The model under review builds one solid part; all positions refer to its coordinate system, in mm. Face numbers are marked on the shaded views. A direction names the side the tool comes from. Round coordinates to 2 decimals unless told otherwise and drop trailing zeros. Write each loop counter-clockwise with the first axis right and the second up, starting at its lowest first coordinate (ties: lowest second). Pieces come first, ordered by that corner, then holes.
Item 1: To check wall thickness, follow L1, parallel to X at y = 1.9, z = 3.5; L2, parallel to X at y = 0.6, z = -4.5; L3, parallel to X at y = 4.4, z = 0. State the ranges of each line that lie inside material, in increasing order.
Item 2: Clearance check with flat-ended pins moving along their axes: pin 1 Ø2 at (y, z) = (2, 6) entering from +X; pin 2 Ø1.5 at (x, y) = (3, 2.5) entering from -Z; pin 3 Ø2 at (x, z) = (0, 10.09) entering from +Y. State where each tip first meets the part, or that it passes through.
Item 3: Add section B-B (y = 3.8). Give the boundary of the cut face in (x, z).
Item 4: Draft analysis for pull direction Z (two halves, no side actions). For the marked faces 3, 4 and 5, state which applies: +Z half, -Z half, draft (parallel to the pull), parting line (faces both ways), or undercut.
Item 5: Machinability: for the marked faces 1 and 2, which of the approach directions +Z, -Z, +X, -X, +Y, -Y give a long, thin tool a straight path to every point of the face, cutting with its end or side? Answer none if there is none.
Item 6: Add section C-C (x = 3.25). Give the boundary of the cut face in (y, z).
Item 7: Add section A-A (x = 8.5). Give the boundary of the cut face in (y, z), plus the area to 3 significant figures.
Item 8: Add section D-D (y = 0.5). State how many separate pieces and enclosed holes the cut face has, plus the area to 3 significant figures.
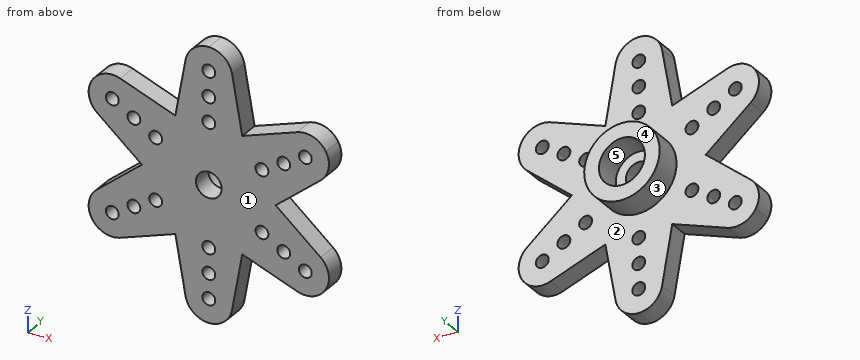
```python
from build123d import *

# Parameters (mm, degrees)
SKETCH1_R           = 15.75
BOSS_EXTRUDE1_DEPTH = 2.35
CUT_EXTRUDE2_START  = -2.35
CUT_EXTRUDE2_DEPTH  = 2.35
SKETCH3_R           = 4.4
SKETCH3_R_2         = 2.68
BOSS_EXTRUDE2_DEPTH = 3.2
SKETCH4_R           = 1.5
CUT_EXTRUDE3_DEPTH  = 22.320518549


with BuildPart() as part:
    # Sketch1 → Boss-Extrude1 (new body)
    with BuildSketch(Plane(origin=(0, 0, 0), x_dir=(1, 0, 0), z_dir=(0, 1, 0))):
        with Locations(Location((0, 0, 0), (0, 0, 270))):
            Circle(SKETCH1_R)
    extrude(amount=BOSS_EXTRUDE1_DEPTH)

    # Sketch2 → Cut-Extrude2 (cut)
    with BuildSketch(Plane(origin=(0, 2.35, 0), x_dir=(1, 0, 0), z_dir=(0, 1, 0)).offset(CUT_EXTRUDE2_START)):
        with BuildLine():
            ThreePointArc((-11.901228971, -6.87117775), (-11.626709919, -5.846658698), (-10.602190866, -6.12117775))
            ThreePointArc((-10.602190866, -6.12117775), (-10.876709919, -7.145696803), (-11.901228971, -6.87117775))
        make_face()
        with BuildLine():
            ThreePointArc((-9.385628943, -5.418795397), (-9.11110989, -4.394276344), (-8.086590837, -4.668795397))
            ThreePointArc((-8.086590837, -4.668795397), (-8.36110989, -5.693314449), (-9.385628943, -5.418795397))
        make_face()
        with BuildLine():
            ThreePointArc((-6.846872878, -3.953043899), (-6.572353825, -2.928524846), (-5.547834772, -3.203043899))
            ThreePointArc((-5.547834772, -3.203043899), (-5.822353825, -4.227562952), (-6.846872878, -3.953043899))
        make_face()
        with BuildLine():
            ThreePointArc((-11.901228971, 6.87117775), (-10.876709919, 7.145696803), (-10.602190866, 6.12117775))
            ThreePointArc((-10.602190866, 6.12117775), (-11.626709919, 5.846658698), (-11.901228971, 6.87117775))
        make_face()
        with BuildLine():
            ThreePointArc((-9.385628943, 5.418795397), (-8.36110989, 5.693314449), (-8.086590837, 4.668795397))
            ThreePointArc((-8.086590837, 4.668795397), (-9.11110989, 4.394276344), (-9.385628943, 5.418795397))
        make_face()
        with BuildLine():
            ThreePointArc((-6.846872878, 3.953043899), (-5.822353825, 4.227562952), (-5.547834772, 3.203043899))
            ThreePointArc((-5.547834772, 3.203043899), (-6.572353825, 2.928524846), (-6.846872878, 3.953043899))
        make_face()
        with BuildLine():
            ThreePointArc((0, 13.742355501), (0.75, 12.992355501), (0, 12.242355501))
            ThreePointArc((0, 12.242355501), (-0.75, 12.992355501), (0, 13.742355501))
        make_face()
        with BuildLine():
            ThreePointArc((0, 7.906087798), (0.75, 7.156087798), (0, 6.406087798))
            ThreePointArc((0, 6.406087798), (-0.75, 7.156087798), (0, 7.906087798))
        make_face()
        with BuildLine():
            ThreePointArc((0, 10.837590793), (0.75, 10.087590793), (0, 9.337590793))
            ThreePointArc((0, 9.337590793), (-0.75, 10.087590793), (0, 10.837590793))
        make_face()
        with BuildLine():
            ThreePointArc((6.846872878, 3.953043899), (6.572353825, 2.928524846), (5.547834772, 3.203043899))
            ThreePointArc((5.547834772, 3.203043899), (5.822353825, 4.227562952), (6.846872878, 3.953043899))
        make_face()
        with BuildLine():
            ThreePointArc((9.385628943, 5.418795397), (9.11110989, 4.394276344), (8.086590837, 4.668795397))
            ThreePointArc((8.086590837, 4.668795397), (8.36110989, 5.693314449), (9.385628943, 5.418795397))
        make_face()
        with BuildLine():
            ThreePointArc((11.901228971, 6.87117775), (11.626709919, 5.846658698), (10.602190866, 6.12117775))
            ThreePointArc((10.602190866, 6.12117775), (10.876709919, 7.145696803), (11.901228971, 6.87117775))
        make_face()
        with BuildLine():
            ThreePointArc((6.846872878, -3.953043899), (5.822353825, -4.227562952), (5.547834772, -3.203043899))
            ThreePointArc((5.547834772, -3.203043899), (6.572353825, -2.928524846), (6.846872878, -3.953043899))
        make_face()
        with BuildLine():
            ThreePointArc((9.385628943, -5.418795397), (8.36110989, -5.693314449), (8.086590837, -4.668795397))
            ThreePointArc((8.086590837, -4.668795397), (9.11110989, -4.394276344), (9.385628943, -5.418795397))
        make_face()
        with BuildLine():
            ThreePointArc((11.901228971, -6.87117775), (10.876709919, -7.145696803), (10.602190866, -6.12117775))
            ThreePointArc((10.602190866, -6.12117775), (11.626709919, -5.846658698), (11.901228971, -6.87117775))
        make_face()
        with BuildLine():
            ThreePointArc((0, -7.906087798), (-0.75, -7.156087798), (0, -6.406087798))
            ThreePointArc((0, -6.406087798), (0.75, -7.156087798), (0, -7.906087798))
        make_face()
        with BuildLine():
            ThreePointArc((0, -10.837590793), (-0.75, -10.087590793), (0, -9.337590793))
            ThreePointArc((0, -9.337590793), (0.75, -10.087590793), (0, -10.837590793))
        make_face()
        with BuildLine():
            ThreePointArc((0, -13.742355501), (-0.75, -12.992355501), (0, -12.242355501))
            ThreePointArc((0, -12.242355501), (0.75, -12.992355501), (0, -13.742355501))
        make_face()
        with BuildLine():
            ThreePointArc((-10.308539952, -9.087515937), (-12.194879886, -9.087515937), (-13.63990011, -7.875))
            ThreePointArc((-13.63990011, -7.875), (-7.875, -13.63990011), (0, -15.75))
            ThreePointArc((0, -15.75), (-1.772579716, -15.104833745), (-2.715749683, -13.471215443))
            Line((-2.715749683, -13.471215443), (-3.9, -6.75499815))
            Line((-3.9, -6.75499815), (-10.308539952, -9.087515937))
        make_face()
        with BuildLine():
            ThreePointArc((-13.024289635, 4.383699506), (-13.967459602, 6.017317808), (-13.63990011, 7.875))
            ThreePointArc((-13.63990011, 7.875), (-15.75, 0), (-13.63990011, -7.875))
            ThreePointArc((-13.63990011, -7.875), (-13.967459602, -6.017317808), (-13.024289635, -4.383699506))
            Line((-13.024289635, -4.383699506), (-7.8, 0))
            Line((-7.8, 0), (-13.024289635, 4.383699506))
        make_face()
        with BuildLine():
            Line((-10.308539952, 9.087515937), (-3.9, 6.75499815))
            Line((-3.9, 6.75499815), (-2.715749683, 13.471215443))
            ThreePointArc((-2.715749683, 13.471215443), (-1.772579716, 15.104833745), (0, 15.75))
            ThreePointArc((0, 15.75), (-7.875, 13.63990011), (-13.63990011, 7.875))
            ThreePointArc((-13.63990011, 7.875), (-12.194879886, 9.087515937), (-10.308539952, 9.087515937))
        make_face()
        with BuildLine():
            ThreePointArc((13.63990011, 7.875), (7.875, 13.63990011), (0, 15.75))
            ThreePointArc((0, 15.75), (1.772579716, 15.104833745), (2.715749683, 13.471215443))
            Line((2.715749683, 13.471215443), (3.9, 6.75499815))
            Line((3.9, 6.75499815), (10.308539952, 9.087515937))
            ThreePointArc((10.308539952, 9.087515937), (12.194879886, 9.087515937), (13.63990011, 7.875))
        make_face()
        with BuildLine():
            ThreePointArc((15.75, 0), (15.213331764, 4.07639996), (13.63990011, 7.875))
            ThreePointArc((13.63990011, 7.875), (13.967459602, 6.017317808), (13.024289635, 4.383699506))
            Line((13.024289635, 4.383699506), (7.8, 0))
            Line((7.8, 0), (13.024289635, -4.383699506))
            ThreePointArc((13.024289635, -4.383699506), (13.967459602, -6.017317808), (13.63990011, -7.875))
            ThreePointArc((13.63990011, -7.875), (15.213331764, -4.07639996), (15.75, 0))
        make_face()
        with BuildLine():
            ThreePointArc((2.715749683, -13.471215443), (1.772579716, -15.104833745), (0, -15.75))
            ThreePointArc((0, -15.75), (7.875, -13.63990011), (13.63990011, -7.875))
            ThreePointArc((13.63990011, -7.875), (12.194879886, -9.087515937), (10.308539952, -9.087515937))
            Line((10.308539952, -9.087515937), (3.9, -6.75499815))
            Line((3.9, -6.75499815), (2.715749683, -13.471215443))
        make_face()
    extrude(amount=CUT_EXTRUDE2_DEPTH, mode=Mode.SUBTRACT)

    # Sketch3 → Boss-Extrude2 (add)
    with BuildSketch(Plane(origin=(0, 2.35, 0), x_dir=(1, 0, 0), z_dir=(0, 1, 0))):
        with Locations(Location((0, 0, 0), (0, 0, 270))):
            Circle(SKETCH3_R)
        with Locations(Location((0, 0, 0), (0, 0, 270))):
            Circle(SKETCH3_R_2, mode=Mode.SUBTRACT)
    extrude(amount=BOSS_EXTRUDE2_DEPTH)

    # Sketch4 → Cut-Extrude3 (cut, through all)
    with BuildSketch(Plane(origin=(0, 2.35, 0), x_dir=(1, 0, 0), z_dir=(0, 1, 0))):
        with Locations(Location((0, 0, 0), (0, 0, 270))):
            Circle(SKETCH4_R)
    extrude(amount=-CUT_EXTRUDE3_DEPTH, mode=Mode.SUBTRACT)


solid = part.part
```
Numbers:
1. L1: x = -11.97 to -6.94, -5.45 to 5.45, 6.94 to 11.97
1. L2: x = -13.15 to -9.25, -8.22 to 8.22, 9.25 to 13.15
1. L3: x = -4.4 to -2.68, 2.68 to 4.4
2. pin 1: stops at x = 14.01
2. pin 2: stops at z = -14.57
2. pin 3: stops at y = 2.35
3. outline: circle Ø8.8 at (0, 0); hole circle Ø5.36 at (0, 0)
4. face 3: parting line
4. face 4: draft
4. face 5: undercut
5. face 1: +Z, -Z, +X, -X, -Y
5. face 2: +Y
6. outline: (0, -10.44) - (2.35, -10.44) - (2.35, -2.97) - (5.55, -2.97) - (5.55, 2.97) - (2.35, 2.97) - (2.35, 10.44) - (0, 10.44) - close
7. outline: (0, -8.43) - (2.35, -8.43) - (2.35, -5.76) - (0, -5.76) - close; (0, -4.33) - (2.35, -4.33) - (2.35, -0.59) - (0, -0.59) - close; (0, 0.59) - (2.35, 0.59) - (2.35, 4.33) - (0, 4.33) - close; (0, 5.76) - (2.35, 5.76) - (2.35, 8.43) - (0, 8.43) - close
7. area: 30.2 mm2
8. separate pieces: 1
8. enclosed holes: 19
8. area: 442 mm2
